Autodesk Inventor part; units mm, degrees
ref_plane "YZ Plane" through (0, 0, 0) normal (1, 0, 0) x (0, 1, 0)
ref_plane "XZ Plane" through (0, 0, 0) normal (0, 1, 0) x (-1, 0, 0)
ref_plane "XY Plane" through (0, 0, 0) normal (0, 0, 1) x (1, 0, 0)
sketch "Sketch1" plane through (0, 0, 0) normal (0, 0, 1) x (1, 0, 0)
  circle A0 centre (-107, 60.0196) radius 2 construction
  circle A1 centre (-27, 60.0196) radius 2 construction
  line L0 (-133, 1) -> (-133, 3) construction
  line L1 (-133, 3) -> (-131, 3) construction
  line L2 (-131, 3) -> (-131, 1) construction
  line L3 (-131, 1) -> (-133, 1) construction
  line L4 (-1, 3) -> (-1, 1) construction
  line L5 (-1, 1) -> (-3, 1) construction
  line L6 (-3, 1) -> (-3, 3) construction
  line L7 (-3, 3) -> (-1, 3) construction
  line L8 (-3, 73) -> (-1, 73) construction
  line L9 (-1, 73) -> (-1, 71) construction
  line L10 (-1, 71) -> (-3, 71) construction
  line L11 (-3, 71) -> (-3, 73) construction
  line L12 (-131, 71) -> (-133, 71) construction
  line L13 (-133, 71) -> (-133, 73) construction
  line L14 (-133, 73) -> (-131, 73) construction
  line L15 (-131, 73) -> (-131, 71) construction
  line L16 (-3, -3) -> (-3, -1) construction
  line L17 (-3, -1) -> (1, -1) construction
  line L18 (1, -1) -> (1, 3) construction
  line L19 (1, 3) -> (3, 3) construction
  line L20 (3, 3) -> (3, 71) construction
  line L21 (3, 71) -> (1, 71) construction
  line L22 (1, 71) -> (1, 75) construction
  line L23 (1, 75) -> (-3, 75) construction
  line L24 (-3, 75) -> (-3, 77) construction
  line L25 (-3, 77) -> (-131, 77) construction
  line L26 (-131, 77) -> (-131, 75) construction
  line L27 (-131, 75) -> (-135, 75) construction
  line L28 (-135, 75) -> (-135, 71) construction
  line L29 (-135, 71) -> (-137, 71) construction
  line L30 (-137, 71) -> (-137, 3) construction
  line L31 (-137, 3) -> (-135, 3) construction
  line L32 (-135, 3) -> (-135, -1) construction
  line L33 (-135, -1) -> (-131, -1) construction
  line L34 (-131, -1) -> (-131, -3) construction
  line L35 (-131, -3) -> (-3, -3) construction
  line L36 (-137, 3) -> (-137, -3) construction
  line L37 (-137, 77) -> (-137, 71) construction
  line L38 (3, -3) -> (-137, -3) construction
  line L39 (-137, -3) -> (-137, 77) construction
  line L40 (-137, 77) -> (3, 77) construction
  line L41 (3, 77) -> (3, -3) construction
  line L42 (7, -7) -> (-141, -7)
  line L43 (-141, -7) -> (-141, 81)
  line L44 (-141, 81) -> (7, 81)
  line L45 (7, 81) -> (7, -7)
  line L46 (3, -3) -> (-3, -3)
  line L47 (-3, -1) -> (-3, -3)
  line L48 (1, -1) -> (1, 3)
  line L49 (3, 3) -> (3, -3)
  line L50 (1, 3) -> (3, 3)
  line L51 (1, -1) -> (-3, -1)
  line L52 (1, 71) -> (3, 71)
  line L53 (3, 71) -> (3, 77)
  line L54 (-3, 77) -> (-3, 75)
  line L55 (1, 75) -> (1, 71)
  line L56 (3, 77) -> (-3, 77)
  line L57 (-3, 75) -> (1, 75)
  line L58 (-131, 77) -> (-131, 75)
  line L59 (-135, 75) -> (-135, 71)
  line L60 (-137, 71) -> (-137, 77)
  line L61 (-131, 77) -> (-137, 77)
  line L62 (-137, 71) -> (-135, 71)
  line L63 (-135, 75) -> (-131, 75)
  line L64 (-131, -3) -> (-131, -1)
  line L65 (-135, -1) -> (-135, 3)
  line L66 (-137, 3) -> (-137, -3)
  line L67 (-131, -3) -> (-137, -3)
  line L68 (-131, -1) -> (-135, -1)
  line L69 (-137, 3) -> (-135, 3)
  line L70 (-1, 1) -> (-3, 1)
  line L71 (-3, 1) -> (-3, 3)
  line L72 (-3, 3) -> (-1, 3)
  line L73 (-1, 3) -> (-1, 1)
  line L74 (-1, 71) -> (-3, 71)
  line L75 (-3, 71) -> (-3, 73)
  line L76 (-3, 73) -> (-1, 73)
  line L77 (-1, 73) -> (-1, 71)
  line L78 (-131, 71) -> (-133, 71)
  line L79 (-133, 71) -> (-133, 73)
  line L80 (-133, 73) -> (-131, 73)
  line L81 (-131, 73) -> (-131, 71)
  line L82 (-131, 1) -> (-133, 1)
  line L83 (-133, 1) -> (-133, 3)
  line L84 (-133, 3) -> (-131, 3)
  line L85 (-131, 3) -> (-131, 1)
  point P0 (0, 0)
  dimension "d0" = 4
extrude "Extrusion1" add sketch "Sketch1" against normal blind 4
sketch "Sketch2" plane through (-141, 81, 0) normal (0, 1, 0) x (1, 0, 0)
  line L0 (148, 0) -> (148, 4)
  line L1 (148, 0) -> (0, 0)
  line L2 (0, 0) -> (0, -2)
  line L3 (0, -2) -> (148, -2)
  line L4 (148, -2) -> (148, 0)
  point P0 (141, 0)
  dimension "d3" = 2
extrude "Extrusion2" add sketch "Sketch2" against normal up to surface (88 mm away)
properties part number "NL_hosuing_Top"
Work out the finished part from the listing and answer in its coordinate system (mm). A direction names the side the tool comes from. Coordinates: 2 decimals unless noted, no trailing zeros. Answer as CSV lines item,"result". Start each with the question number.
Item 1: Determine the mould class of faces 3 (the face through (-66, -7, -1)), 4 (the face through (-68, 81, -1)), 5 (the face through (-134, -3, -2)) for opening direction Y: released by +Y, released by -Y, zero draft, split by the parting line, or undercut.
Item 2: A tool of negligible diameter and unlimited length cuts with its end or side. For faces 1 (the face through (7, 38, -1)), 2 (the face through (-135, 1, -2)), from which of +Z, -Z, +X, -X, +Y, -Y can it reach the whole face along a straight path? Write none if from no direction.
Item 3: Consider L1, parallel to X at y = 2, z = -2.6; L2, parallel to X at y = 73.5, z = -3.5. Determine where each line is inside the solid, lowest interval first.
Checks:
1,face 3,"released by -Y"
1,face 4,"released by +Y"
1,face 5,"undercut"
2,face 1,"+Z, -Z, +X, +Y, -Y"
2,face 2,"-Z"
3,L1,"x = -141 to -137, -135 to -133, -131 to -3, -1 to 1, 3 to 7"
3,L2,"x = -141 to -137, -135 to 1, 3 to 7"
